Design review of the part shown in the three views and the two pictorial views. Dimensions are in mm from the part's minimum x, y and z. A direction names the side the tool comes from. Round coordinates to 2 decimals unless told otherwise and drop trailing zeros. Loops run counter-clockwise (first coordinate to the right, second up) from the corner with the lowest first, then second, coordinate; pieces in that order, holes last.
1. Tool access review of the marked faces 1, 2 and 3: name each direction out of +Z, -Z, +X, -X, +Y, -Y from which nothing blocks a thin tool from reaching the whole face with its end or side.
2. Consider section C-C on z = 25. State the section outline as (x, y) points, then the cut area to 3 significant figures.
3. To check wall thickness, follow line 1 along Y through (x, z) = (13.75, 25.75); line 2 along Z through (x, y) = (10, 17.95); line 3 along X through (y, z) = (18, 21). State the ranges of each line that lie inside material, in increasing order.
4. Consider section D-D on y = 2. State the section outline as (x, z) points.
5. Consider section B-B on z = 17.75. State the section outline as (x, y) points.
6. Clearance check with flat-ended pins moving along their axes: pin 1 Ø2 at (y, z) = (13, 5.5) entering from -X; pin 2 Ø4.5 at (x, z) = (10, 25) entering from -Y; pin 3 Ø2.5 at (x, z) = (18.5, 11.5) entering from +Y; pin 4 Ø4 at (y, z) = (9, 20) entering from +X. State where each tip first meets the part, or that it passes through.
7. Consider section A-A on x = 11.5. State the section outline as (y, z) points, then the cut area to 3 significant figures.
8. Draft analysis for pull direction X (two halves, no side actions). For the marked faces 4, 5, 6 and 7, state which applies: released by +X, released by -X, zero draft, split by the parting line, or undercut.
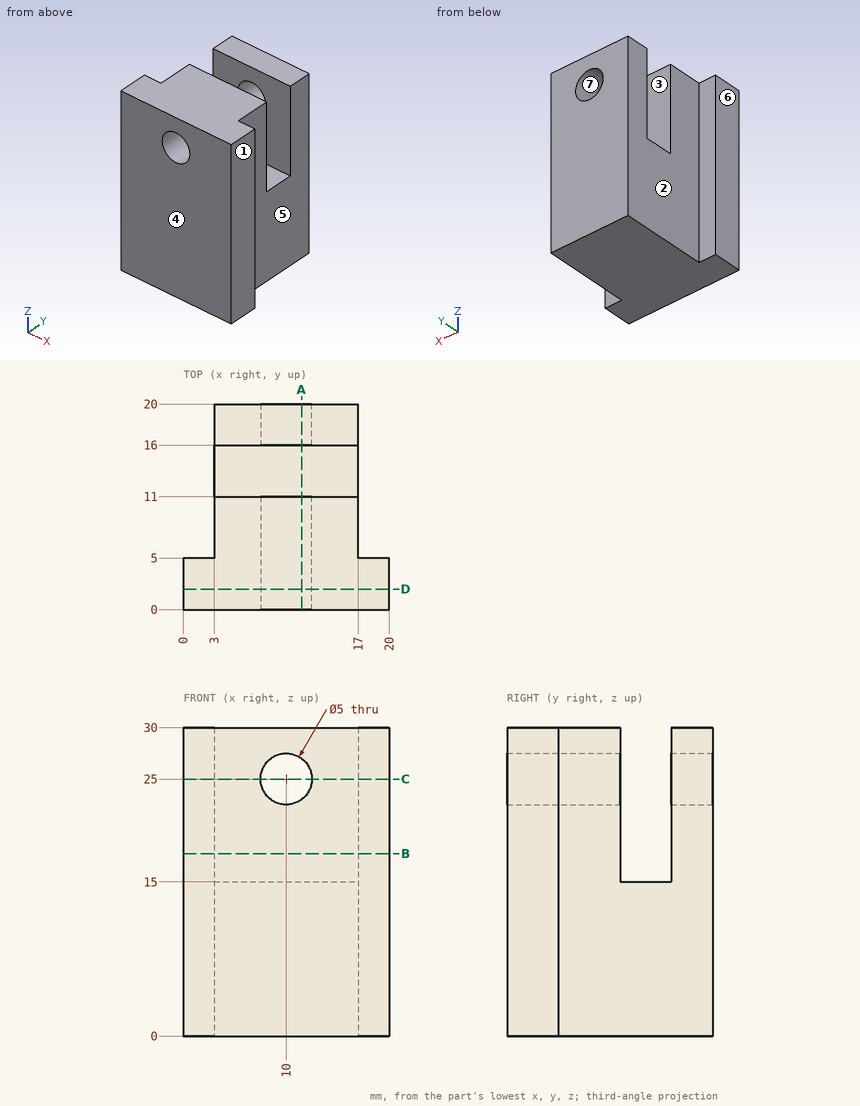
Resolved:
1. face 1: +Z, -Z, +X, +Y, -Y
1. face 2: +Z, -Z, -X, +Y
1. face 3: +Z, +X, -X
2. outline: (0, 0) - (7.5, 0) - (7.5, 11) - (3, 11) - (3, 5) - (0, 5) - close; (3, 16) - (7.5, 16) - (7.5, 20) - (3, 20) - close; (12.5, 0) - (20, 0) - (20, 5) - (17, 5) - (17, 11) - (12.5, 11) - close; (12.5, 16) - (17, 16) - (17, 20) - (12.5, 20) - close
2. area: 165 mm2
3. line 1: y = 0 to 11, 16 to 20
3. line 2: z = 0 to 22.5, 27.5 to 30
3. line 3: x = 3 to 17
4. outline: (0, 0) - (20, 0) - (20, 30) - (0, 30) - close; hole circle Ø5 at (10, 25)
5. outline: (0, 0) - (20, 0) - (20, 5) - (17, 5) - (17, 11) - (3, 11) - (3, 5) - (0, 5) - close; (3, 16) - (17, 16) - (17, 20) - (3, 20) - close
6. pin 1: stops at x = 3
6. pin 2: passes through
6. pin 3: stops at y = 5
6. pin 4: stops at x = 17
7. outline: (0, 0) - (20, 0) - (20, 23) - (16, 23) - (16, 15) - (11, 15) - (11, 23) - (0, 23) - close; (0, 27) - (11, 27) - (11, 30) - (0, 30) - close; (16, 27) - (20, 27) - (20, 30) - (16, 30) - close
7. area: 465 mm2
8. face 4: zero draft
8. face 5: released by +X
8. face 6: released by -X
8. face 7: undercut
